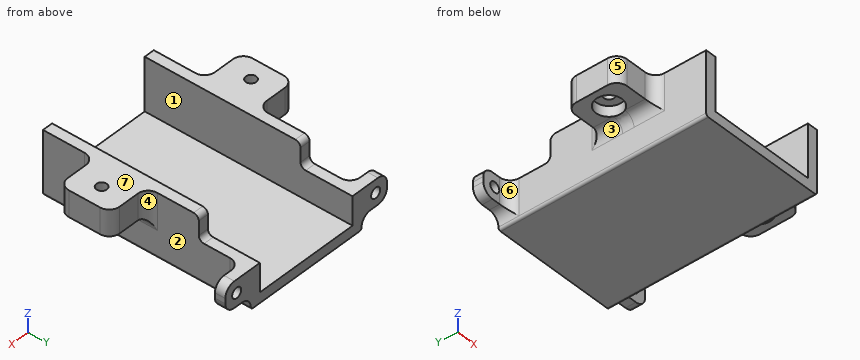
```python
from build123d import *

# Parameters (mm, degrees)
BOSS_EXTRUDE1_DEPTH = 101.6
SKETCH2_W           = 25.4
SKETCH2_H           = 25.4
BOSS_EXTRUDE2_DEPTH = 12.7
SKETCH3_R           = 2.54
CUT_EXTRUDE1_DEPTH  = 116.280188272
SKETCH4_R           = 6.35
CUT_EXTRUDE2_DEPTH  = 5.08
FILLET1_R           = 5.08
SKETCH5_W           = 14.224
SKETCH5_H           = 12.7
SKETCH5_R           = 2.54
BOSS_EXTRUDE3_DEPTH = 5.08
FILLET2_R           = 5.08
FILLET3_R           = 5.08
SKETCH6_W           = 11.938
SKETCH6_H           = 25.4
CUT_EXTRUDE3_DEPTH  = 132.986426559
FILLET4_R           = 2.54
FILLET5_R           = 1.27


with BuildPart() as part:
    # Sketch1 → Boss-Extrude1 (new body)
    with BuildSketch(Plane(origin=(0, 0, 0), x_dir=(1, 0, 0), z_dir=(0, 1, 0))):
        Polygon((-25.908, -12.954), (-25.908, 12.954), (25.908, 12.954), (25.908, -12.954), (30.988, -12.954), (30.988, 18.034), (-30.988, 18.034), (-30.988, -12.954), align=None)
    extrude(amount=BOSS_EXTRUDE1_DEPTH)

    # Sketch2 → Boss-Extrude2 (add)
    with BuildSketch(Plane.XY.offset(12.954)):
        with Locations((38.608, 38.1)):
            Rectangle(SKETCH2_W, SKETCH2_H)
        with Locations((-38.608, 38.1)):
            Rectangle(SKETCH2_W, SKETCH2_H)
    extrude(amount=-BOSS_EXTRUDE2_DEPTH)

    # Sketch3 → Cut-Extrude1 (cut, through all)
    with BuildSketch(Plane(origin=(0, 0, 0.254), x_dir=(-1, 0, 0), z_dir=(0, 0, -1))):
        with Locations((-41.783, 38.1)):
            Circle(SKETCH3_R)
        with Locations(Location((41.783, 38.1, 0), (0, 0, 180))):
            Circle(SKETCH3_R)
    extrude(amount=-CUT_EXTRUDE1_DEPTH, mode=Mode.SUBTRACT)

    # Sketch4 → Cut-Extrude2 (cut)
    with BuildSketch(Plane(origin=(0, 0, 0.254), x_dir=(-1, 0, 0), z_dir=(0, 0, -1))):
        with Locations((-41.783, 38.1)):
            Circle(SKETCH4_R)
        with Locations((41.783, 38.1)):
            Circle(SKETCH4_R)
    extrude(amount=-CUT_EXTRUDE2_DEPTH, mode=Mode.SUBTRACT)

    # Fillet1
    fillet1_edges = [part.edges().sort_by_distance(p)[0] for p in [
        (51.308, 25.4, 6.604),
        (30.988, 50.8, 6.604),
        (51.308, 50.8, 6.604),
        (30.988, 25.4, 6.604),
        (30.988, 38.1, 0.254),
        (-30.988, 25.4, 6.604),
        (-51.308, 25.4, 6.604),
        (-30.988, 50.8, 6.604),
        (-51.308, 50.8, 6.604),
        (-30.988, 38.1, 0.254),
    ]]
    fillet(fillet1_edges, radius=FILLET1_R)

    # Sketch5 → Boss-Extrude3 (add)
    # profile 1 of 2: a face of its own
    with BuildSketch(Plane(origin=(0, 101.6, 0), x_dir=(1, 0, 0), z_dir=(0, 1, 0))):
        with Locations((38.1, 5.334)):
            Rectangle(SKETCH5_W, SKETCH5_H)
        with Locations(Location((38.862, 5.334, 0), (0, 0, 270))):
            Circle(SKETCH5_R, mode=Mode.SUBTRACT)
    # profile 2 of 2: a face of its own
    with BuildSketch(Plane(origin=(0, 101.6, 0), x_dir=(1, 0, 0), z_dir=(0, 1, 0))):
        with Locations((-38.1, 5.334)):
            Rectangle(SKETCH5_W, SKETCH5_H)
        with Locations(Location((-38.862, 5.334, 0), (0, 0, 270))):
            Circle(SKETCH5_R, mode=Mode.SUBTRACT)
    extrude(amount=-BOSS_EXTRUDE3_DEPTH)

    # Fillet2
    fillet2_edges = [part.edges().sort_by_distance(p)[0] for p in [
        (-30.988, 99.06, -11.684),
        (-30.988, 96.52, -5.334),
        (30.988, 99.06, -11.684),
        (30.988, 96.52, -5.334),
    ]]
    fillet(fillet2_edges, radius=FILLET2_R)

    # Fillet3
    fillet3_edges = [part.edges().sort_by_distance(p)[0] for p in [
        (-45.212, 99.06, -11.684),
        (-45.212, 99.06, 1.016),
        (45.212, 99.06, -11.684),
        (45.212, 99.06, 1.016),
    ]]
    fillet(fillet3_edges, radius=FILLET3_R)

    # Sketch6 → Cut-Extrude3 (cut, through all)
    with BuildSketch(Plane.ZY.offset(30.988)):
        with Locations((6.985, 88.9)):
            Rectangle(SKETCH6_W, SKETCH6_H)
    extrude(amount=-CUT_EXTRUDE3_DEPTH, mode=Mode.SUBTRACT)

    # Fillet4
    fillet4_edges = [part.edges().sort_by_distance(p)[0] for p in [
        (28.448, 76.2, 12.954),
        (28.448, 76.2, 1.016),
        (-28.448, 76.2, 1.016),
        (-28.448, 76.2, 12.954),
    ]]
    fillet(fillet4_edges, radius=FILLET4_R)

    # Fillet5
    fillet5_edges = [part.edges().sort_by_distance(p)[0] for p in [
        (30.988, 50.8, -18.034),
        (-30.988, 50.8, -18.034),
    ]]
    fillet(fillet5_edges, radius=FILLET5_R - 0.0001)  # a hair under: the kernel refuses the full size


solid = part.part
```
Could you check a few things on this model? Use its own coordinates, in mm. Face numbers are marked on the shaded views. A direction names the side the tool comes from. Round coordinates to 2 decimals unless told otherwise and drop trailing zeros. Loops run counter-clockwise (first coordinate to the right, second up) from the corner with the lowest first, then second, coordinate; pieces in that order, holes last. Notation, with made-up numbers: (47, 55.5) - (102, 55.5) arc R7 ccw to (102, 68.5) - close; hole circle Ø6 at (-26, 68). An arc over 180 degrees is marked (long way). Answer in a Markdown table with one row per item. Add a question column.
(1) I'm going to push flat-ended pins straight in: pin 1 (10 mm diameter, centred on x = -40.5, z = -4, fed in from -Y); pin 2 (6 mm diameter, centred on x = -38.862, z = -5.334, fed in from -Y); pin 3 (10 mm diameter, centred on x = 44, y = 37.5, fed in from -Z). Where does each tip first touch, or does it pass through?
(2) If we section it at D-D (y = 54): Please give me the cut outline in (x, z), plus the area to 3 significant figures.
(3) I need wall thicknesses on line 1 along X through (y, z) = (38, 11); line 2 along X through (y, z) = (38, 1); line 3 along X through (y, z) = (32, 7). Which ranges of each line are inside material? Lowest first, please.
(4) If we section it at C-C (x = -3.5): Please give me the cut outline in (y, z).
(5) If we section it at B-B (y = 33): Please give me the cut outline in (x, z).
(6) For the marked faces 1, 2 and 3, which set-ups out of +Z, -Z, +X, -X, +Y, -Y let a thin tool reach every point of the face, with its end or its side?
(7) If we mould it in two halves opening along Y, with no side actions, what happens to the marked faces 4, 5, 6 and 7? For each: pulls with the +Y half, pulls with the -Y half, needs draft (parallel to the pull), parting line crosses it, or undercut.
(8) If we section it at A-A (z = -10): Please give me the cut outline in (x, y), plus the area to 3 significant figures.
Model answer:
| question | item | result |
|---|---|---|
| 1 | pin 1 | stops at y = 25.4 |
| 1 | pin 2 | stops at y = 96.52 |
| 1 | pin 3 | stops at z = 0.25 |
| 2 | outline | (-31.35, -2.95) arc R5.08 cw to (-30.99, -4.83) - (-30.99, -16.76) arc R1.27 ccw to (-29.72, -18.03) - (29.72, -18.03) arc R1.27 ccw to (30.99, -16.76) - (30.99, -4.83) arc R5.08 cw to (31.35, -2.95) - (31.35, 12.95) - (25.91, 12.95) - (25.91, -12.95) - (-25.91, -12.95) - (-25.91, 12.95) - (-31.35, 12.95) - close |
| 2 | area | 589 mm² |
| 3 | line 1 | x = -51.31 to -44.32, -39.24 to -25.91, 25.91 to 39.24, 44.32 to 51.31 |
| 3 | line 2 | x = -51.31 to -48.13, -35.43 to -25.91, 25.91 to 35.43, 48.13 to 51.31 |
| 3 | line 3 | x = -51.31 to -25.91, 25.91 to 51.31 |
| 4 | outline | (0, -18.03) - (101.6, -18.03) - (101.6, -12.95) - (0, -12.95) - close |
| 5 | outline | (-51.31, 0.25) - (-45.57, 0.25) - (-45.57, 5.33) - (-38, 5.33) - (-38, 0.25) - (-36.07, 0.25) arc R5.08 cw to (-30.99, -4.83) - (-30.99, -16.76) arc R1.27 ccw to (-29.72, -18.03) - (29.72, -18.03) arc R1.27 ccw to (30.99, -16.76) - (30.99, -4.83) arc R5.08 cw to (36.07, 0.25) - (38, 0.25) - (38, 5.33) - (45.57, 5.33) - (45.57, 0.25) - (51.31, 0.25) - (51.31, 12.95) - (25.91, 12.95) - (25.91, -12.95) - (-25.91, -12.95) - (-25.91, 12.95) - (-51.31, 12.95) - close |
| 6 | face 1 | +Z, +Y, -Y |
| 6 | face 2 | -Z, +X |
| 6 | face 3 | -Z, -X, -Y |
| 7 | face 4 | undercut |
| 7 | face 5 | pulls with the -Y half |
| 7 | face 6 | undercut |
| 7 | face 7 | needs draft |
| 8 | outline | (-43.91, 96.52) - (-36.07, 96.52) arc R5.08 cw to (-30.99, 91.44) - (-30.99, 0) - (-25.91, 0) - (-25.91, 101.6) - (-43.91, 101.6) - close; (25.91, 0) - (30.99, 0) - (30.99, 91.44) arc R5.08 cw to (36.07, 96.52) - (43.91, 96.52) - (43.91, 101.6) - (25.91, 101.6) - close |
| 8 | area | 1,170 mm² |
